Source: CAD feature listing. Evaluate the final solid. Frame: model axes, mm. Face numbers are marked on the shaded views. A direction names the side the tool comes from. Round coordinates to 2 decimals unless told otherwise and drop trailing zeros. Order: outer loops, then holes, each group sorted by start corner. A loop starts at its lowest first (then second) coordinate and runs counter-clockwise, first axis right, second up. Notation, with made-up numbers: (-40, 81.25) -> (-28, 81.25) arc R28 cw to (-28, 114.25) -> close; hole circle Ø11 at (-35, 55). An arc over 180 degrees is marked (long way). Answer as CSV lines item,"result".
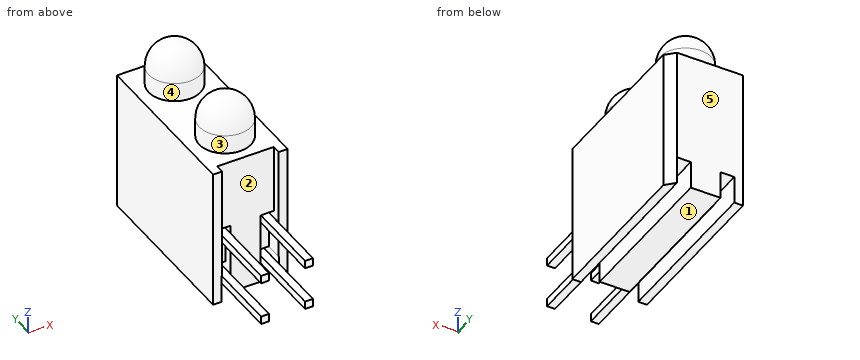
from build123d import *

# Parameters (mm, degrees)
EXTRUSION1_DEPTH   = 8.13
ESQUISSE2_W        = 0.8
ESQUISSE2_H        = 1.6
EXTRUSION2_DEPTH   = 10.55
ESQUISSE4_W        = 0.78
ESQUISSE4_H        = 2.54
EXTRUSION3_DEPTH   = 0.5
ESQUISSE5_W        = 0.46
ESQUISSE5_H        = 0.46
EXTRUSION4_DEPTH   = 4.68
ESQUISSE6_W        = 0.46
ESQUISSE6_H        = 0.46
EXTRUSION5_DEPTH   = 11.53
EXTRUSION5_2_DEPTH = 11.53
ESQUISSE7_W        = 0.46
ESQUISSE7_H        = 0.46
EXTRUSION6_DEPTH   = 0.22


with BuildPart() as part:
    # Esquisse1 → Extrusion1 (new body)
    with BuildSketch(Plane.XY):
        Polygon((-3.8, 0), (-3.8, 0.5), (-0.52, 0.5), (-0.52, 0), (0, 0), (0, 9.15), (-0.5, 9.65), (-4.32, 9.65), (-4.32, 0), align=None)
    extrude(amount=EXTRUSION1_DEPTH)

    # Esquisse2 → Extrusion2 (cut)
    with BuildSketch(Plane(origin=(0, 9.65, 0), x_dir=(1, 0, 0), z_dir=(0, 1, 0))):
        with Locations((-0.9, -0.8)):
            Rectangle(ESQUISSE2_W, ESQUISSE2_H)
        with Locations((-3.42, -0.8)):
            Rectangle(ESQUISSE2_W, ESQUISSE2_H)
    extrude(amount=-EXTRUSION2_DEPTH, mode=Mode.SUBTRACT)

    # Esquisse4 → Extrusion3 (cut)
    with BuildSketch(Plane.XZ.offset(-0.5)):
        with Locations((-3.41, 2.87)):
            Rectangle(ESQUISSE4_W, ESQUISSE4_H)
        with Locations((-0.91, 2.87)):
            Rectangle(ESQUISSE4_W, ESQUISSE4_H)
    extrude(amount=-EXTRUSION3_DEPTH, mode=Mode.SUBTRACT)

    # Esquisse5 → Extrusion4 (add)
    with BuildSketch(Plane.XZ.offset(3.68)):
        with Locations((-3.43, 3.69)):
            Rectangle(ESQUISSE5_W, ESQUISSE5_H)
        with Locations((-0.89, 3.69)):
            Rectangle(ESQUISSE5_W, ESQUISSE5_H)
    extrude(amount=-EXTRUSION4_DEPTH)



with BuildPart() as body_2:
    # Esquisse6 → Extrusion5 (new body)
    with BuildSketch(Plane.XZ.offset(3.68)):
        with Locations((-3.43, 1.15)):
            Rectangle(ESQUISSE6_W, ESQUISSE6_H)
    extrude(amount=-EXTRUSION5_DEPTH)


with BuildPart() as body_3:
    # Esquisse6 → Extrusion5 2 (new body)
    with BuildSketch(Plane.XZ.offset(3.68)):
        with Locations((-0.89, 1.15)):
            Rectangle(ESQUISSE6_W, ESQUISSE6_H)
    extrude(amount=-EXTRUSION5_2_DEPTH)


with BuildPart() as part_1:
    add(part.part)

    add(body_2.part)  # Extrusion6 merges body 2

    add(body_3.part)  # Extrusion6 merges body 3
    # Esquisse7 → Extrusion6 (add)
    with BuildSketch(Plane.XY.offset(1.38)):
        with Locations((-0.89, 7.62)):
            Rectangle(ESQUISSE7_W, ESQUISSE7_H)
        with Locations((-3.43, 7.62)):
            Rectangle(ESQUISSE7_W, ESQUISSE7_H)
    extrude(amount=EXTRUSION6_DEPTH)

    # Esquisse9 → Révolution1 (revolve)
    with BuildSketch(Plane(origin=(-2.16, 0, 0), x_dir=(0, 0, -1), z_dir=(1, 0, 0))):
        with BuildLine():
            Line((-9.23, 1.04), (-8.13, 1.04))
            Line((-8.13, 1.04), (-8.13, 2.54))
            Line((-8.13, 2.54), (-10.73, 2.54))
            ThreePointArc((-10.73, 2.54), (-10.290660172, 1.479339828), (-9.23, 1.04))
        make_face()
    revolve(axis=Axis((-2.16, 2.54, 13.741236879), (0, 0, -1)))

    # Esquisse10 → Révolution2 (revolve)
    with BuildSketch(Plane(origin=(-2.16, 0, 0), x_dir=(0, 0, -1), z_dir=(1, 0, 0))):
        with BuildLine():
            Line((-9.23, 6.12), (-8.13, 6.12))
            Line((-8.13, 6.12), (-8.13, 7.62))
            Line((-8.13, 7.62), (-10.73, 7.62))
            ThreePointArc((-10.73, 7.62), (-10.290660172, 6.559339828), (-9.23, 6.12))
        make_face()
    revolve(axis=Axis((-2.16, 7.62, 13.129927016), (0, 0, -1)))


solid = part_1.part
1. Line query: L1, parallel to X at y = 6.25, z = 0.5; L2, parallel to X at y = -1.5, z = 1.25; L3, parallel to Z at x = -3.2, y = 9. Output: solid intervals per line, ascending. Write a range as [from, to].
Results below:
L1,"[-4.32, -3.82], [-3.02, -1.3], [-0.5, 0]"
L2,"[-3.66, -3.2], [-1.12, -0.66]"
L3,"[1.6, 8.13]"
2. Mould query, pull axis Y, two halves, no side actions, for the marked faces 1, 2 and 3. Classes: released by +Y, released by -Y, zero draft, split by the parting line, or undercut.
Results below:
face 1,"zero draft"
face 2,"released by -Y"
face 3,"undercut"
3. Section query A-A on y = -0.25. Return loops of the section in (x, z).
Results below:
outline,"(-3.66, 0.92) -> (-3.2, 0.92) -> (-3.2, 1.38) -> (-3.66, 1.38) -> close; (-3.66, 3.46) -> (-3.2, 3.46) -> (-3.2, 3.92) -> (-3.66, 3.92) -> close; (-1.12, 0.92) -> (-0.66, 0.92) -> (-0.66, 1.38) -> (-1.12, 1.38) -> close; (-1.12, 3.46) -> (-0.66, 3.46) -> (-0.66, 3.92) -> (-1.12, 3.92) -> close"
4. Pin query (flat end, axial travel): pin 1 (2.5 mm diameter, centred on x = -2.5, z = 6, fed in from -Y); pin 2 (2 mm diameter, centred on x = -0.5, y = 7, fed in from +Z); pin 3 (0.7 mm diameter, centred on y = -0.5, z = 1, fed in from +X). Return the tip coordinate at first contact, or that it passes through.
Results below:
pin 1,"y = 0.5"
pin 2,"z = 10.52"
pin 3,"x = -0.66"
5. Reachability of the marked faces 4 and 5 from +Z, -Z, +X, -X, +Y, -Y: full face, straight path, thin tool, end or side. Return the list, or none.
Results below:
face 4,"+Z"
face 5,"+Z, -Z, +X, -X, +Y"
6. Section query D-D on z = 8.75. Return loops of the section in (x, y), and give its area (3 significant figures).
Results below:
outline,"circle Ø3 at (-2.16, 2.54); circle Ø3 at (-2.16, 7.62)"
area,"14.1 mm2"
7. Section query B-B on x = -2.16. Return loops of the section in (y, z).
Results below:
outline,"(0.5, 0) -> (9.65, 0) -> (9.65, 8.13) -> (9.12, 8.13) -> (9.12, 9.23) arc R1.5 ccw to (6.12, 9.23) -> (6.12, 8.13) -> (4.04, 8.13) -> (4.04, 9.23) arc R1.5 ccw to (1.04, 9.23) -> (1.04, 8.13) -> (0.5, 8.13) -> close"
8. Section query C-C on y = 4.25. Return loops of the section in (x, z).
Results below:
outline,"(-4.32, 0) -> (-3.82, 0) -> (-3.82, 1.6) -> (-3.02, 1.6) -> (-3.02, 0) -> (-1.3, 0) -> (-1.3, 1.6) -> (-0.5, 1.6) -> (-0.5, 0) -> (0, 0) -> (0, 8.13) -> (-4.32, 8.13) -> close; (-3.66, 0.92) -> (-3.2, 0.92) -> (-3.2, 1.38) -> (-3.66, 1.38) -> close; (-1.12, 0.92) -> (-0.66, 0.92) -> (-0.66, 1.38) -> (-1.12, 1.38) -> close"
